Design review of the part built by this model. Coordinates are the model's own, in mm. Face numbers are marked on the shaded views. A direction names the side the tool comes from. Round coordinates to 2 decimals unless told otherwise and drop trailing zeros. Order: outer loops, then holes, each group sorted by start corner. A loop starts at its lowest first (then second) coordinate and runs counter-clockwise, first axis right, second up. Notation, with made-up numbers: (55, 56.5) - (66, 56.5) arc R23 ccw to (66, 91.5) - close; hole circle Ø3 at (42.5, 83.5). An arc over 180 degrees is marked (long way). Use CSV: the item, a comma, the result in double quotes.
from build123d import *

# Parameters (mm, degrees)
SKETCH1_W           = 105
SKETCH1_H           = 70
BOSS_EXTRUDE1_DEPTH = 10
SKETCH2_W           = 20
SKETCH2_H           = 70
BOSS_EXTRUDE2_DEPTH = 70
CUT_EXTRUDE1_DEPTH  = 20
SKETCH4_R           = 25.5
CUT_EXTRUDE2_DEPTH  = 10
SKETCH5_R           = 15.5
CUT_EXTRUDE3_DEPTH  = 4
SKETCH7_R           = 2.5
CUT_EXTRUDE5_DEPTH  = 10
SKETCH9_W           = 10
SKETCH9_H           = 70
BOSS_EXTRUDE4_DEPTH = 35
SKETCH10_R          = 19
CUT_EXTRUDE7_DEPTH  = 10
SKETCH11_R          = 2.5
CUT_EXTRUDE9_DEPTH  = 10
SKETCH6_R           = 12.5
CUT_EXTRUDE10_DEPTH = 10
SKETCH13_W          = 35
SKETCH13_H          = 35
CUT_EXTRUDE11_DEPTH = 10


with BuildPart() as part:
    # Sketch1 → Boss-Extrude1 (new body)
    with BuildSketch(Plane(origin=(0, 0, 0), x_dir=(1, 0, 0), z_dir=(0, 1, 0))):
        Rectangle(SKETCH1_W, SKETCH1_H)
    extrude(amount=BOSS_EXTRUDE1_DEPTH)

    # Sketch2 → Boss-Extrude2 (add)
    with BuildSketch(Plane(origin=(0, 10, 0), x_dir=(1, 0, 0), z_dir=(0, 1, 0))):
        with Locations((42.5, 0)):
            Rectangle(SKETCH2_W, SKETCH2_H)
    extrude(amount=BOSS_EXTRUDE2_DEPTH)

    # Sketch3 → Cut-Extrude1 (cut)
    with BuildSketch(Plane.ZY.offset(-32.5)):
        with BuildLine():
            Line((3e-08, 80), (-35, 80))
            Line((-35, 80), (-35, 45))
            ThreePointArc((-35, 45), (-24.748737331, 69.748737352), (3e-08, 80))
        make_face()
        with BuildLine():
            Line((35, 80), (3e-08, 80))
            ThreePointArc((3e-08, 80), (24.748737352, 69.748737331), (35, 45))
            Line((35, 45), (35, 80))
        make_face()
    extrude(amount=-CUT_EXTRUDE1_DEPTH, mode=Mode.SUBTRACT)

    # Sketch4 → Cut-Extrude2 (cut)
    with BuildSketch(Plane.ZY.offset(-32.5)):
        with Locations((0, 45)):
            Circle(SKETCH4_R)
    extrude(amount=-CUT_EXTRUDE2_DEPTH, mode=Mode.SUBTRACT)

    # Sketch5 → Cut-Extrude3 (cut)
    with BuildSketch(Plane.ZY.offset(-42.5)):
        with Locations((0, 45)):
            Circle(SKETCH5_R)
    extrude(amount=-CUT_EXTRUDE3_DEPTH, mode=Mode.SUBTRACT)

    # Sketch7 → Cut-Extrude5 (cut)
    with BuildSketch(Plane.ZY.offset(-42.5)):
        with Locations((14.142135624, 59.142135624)):
            Circle(SKETCH7_R)
        with Locations((14.142135624, 30.857864376)):
            Circle(SKETCH7_R)
        with Locations((-14.142135624, 30.857864376)):
            Circle(SKETCH7_R)
        with Locations((-14.142135624, 59.142135624)):
            Circle(SKETCH7_R)
    extrude(amount=-CUT_EXTRUDE5_DEPTH, mode=Mode.SUBTRACT)

    # Sketch9 → Boss-Extrude4 (add)
    with BuildSketch(Plane(origin=(0, 10, 0), x_dir=(1, 0, 0), z_dir=(0, 1, 0))):
        with Locations((-47.5, 0)):
            Rectangle(SKETCH9_W, SKETCH9_H)
    extrude(amount=BOSS_EXTRUDE4_DEPTH)

    # Sketch10 → Cut-Extrude7 (cut)
    with BuildSketch(Plane.ZY.offset(52.5)):
        with Locations((0, 45)):
            Circle(SKETCH10_R)
    extrude(amount=-CUT_EXTRUDE7_DEPTH, mode=Mode.SUBTRACT)

    # Sketch11 → Cut-Extrude9 (cut)
    with BuildSketch(Plane(origin=(0, 10, 0), x_dir=(1, 0, 0), z_dir=(0, 1, 0))):
        with Locations((-32.5, 25)):
            Circle(SKETCH11_R)
        with Locations((22.5, 25)):
            Circle(SKETCH11_R)
        with Locations((22.5, -25)):
            Circle(SKETCH11_R)
        with Locations((-32.5, -25)):
            Circle(SKETCH11_R)
    extrude(amount=-CUT_EXTRUDE9_DEPTH, mode=Mode.SUBTRACT)

    # Sketch6 → Cut-Extrude10 (cut)
    with BuildSketch(Plane.ZY.offset(-46.5)):
        with Locations((0, 45)):
            Circle(SKETCH6_R)
    extrude(amount=-CUT_EXTRUDE10_DEPTH, mode=Mode.SUBTRACT)

    # Sketch13 → Cut-Extrude11 (cut)
    with BuildSketch(Plane(origin=(0, 10, 0), x_dir=(1, 0, 0), z_dir=(0, 1, 0))):
        with Locations((-5, 0)):
            Rectangle(SKETCH13_W, SKETCH13_H)
    extrude(amount=-CUT_EXTRUDE11_DEPTH, mode=Mode.SUBTRACT)


solid = part.part
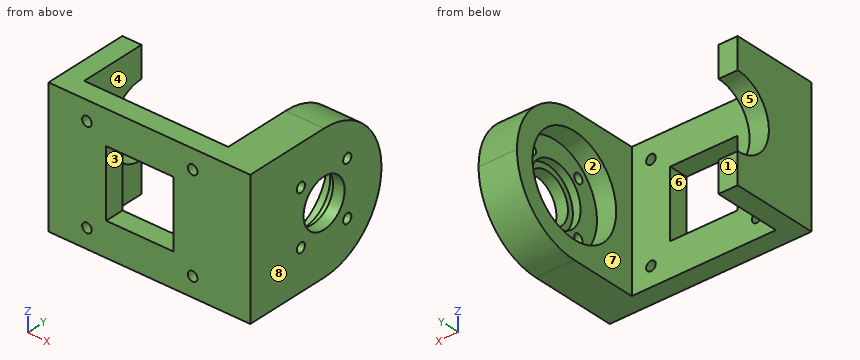
1) We need section B-B (x = -32.5). Give the boundary of the cut face in (y, z), then the cut area to 3 significant figures.
Data:
outline,"(0, -35) - (10, -35) - (10, -27.5) - (0, -27.5) - close; (0, -22.5) - (10, -22.5) - (10, 22.5) - (0, 22.5) - close; (0, 27.5) - (10, 27.5) - (10, 35) - (0, 35) - close"
area,"600 mm2"
2) Insertion check: pin 1 Ø1 at (x, z) = (22.5, 13) entering from +Y; pin 2 Ø15.5 at (y, z) = (37.5, -2.5) entering from -X; pin 3 Ø8 at (x, z) = (-50, -30.5) entering from +Y. Each pin has a flat end and moves straight along its axis. Give the tip position at first contact, or say it passes through.
Data:
pin 1,"stops at y = 10"
pin 2,"stops at x = 42.5"
pin 3,"stops at y = 45"
3) For the marked faces 1, 2, 3 and 4, list the 3-axis set-ups (+Z, -Z, +X, -X, +Y, -Y) from which the entire face can be reached by the end or side of a thin tool; tool diameter is ignored.
Data:
face 1,"+Z, -Z, -X, +Y"
face 2,"none"
face 3,"+Y, -Y"
face 4,"+Z, -Z, +Y"
4) We need section A-A (x = -18). Give the boundary of the cut face in (y, z).
Data:
outline,"(0, -35) - (10, -35) - (10, -17.5) - (0, -17.5) - close; (0, 17.5) - (10, 17.5) - (10, 35) - (0, 35) - close"
5) To check wall thickness, follow L1, parallel to X at y = 7.25, z = -25; L2, parallel to X at y = 9, z = 8; L3, parallel to X at y = 36, z = -25. State the ranges of each line that lie inside material, in increasing order. Write a range as from..to.
Data:
L1,"x = -52.5..-35, -30..20, 25..52.5"
L2,"x = -52.5..-22.5, 12.5..52.5"
L3,"x = -52.5..-42.5, 32.5..52.5"
6) We need section D-D (y = 40.5). Give the boundary of the cut face in (x, z).
Data:
outline,"(-52.5, -35) - (-42.5, -35) - (-42.5, -18.46) - (-52.5, -18.46) - close; (-52.5, 18.46) - (-42.5, 18.46) - (-42.5, 35) - (-52.5, 35) - close; (32.5, -35) - (52.5, -35) - (52.5, -11.66) - (46.5, -11.66) - (46.5, -14.83) - (42.5, -14.83) - (42.5, -25.1) - (32.5, -25.1) - close; (32.5, 25.1) - (42.5, 25.1) - (42.5, 14.83) - (46.5, 14.83) - (46.5, 11.66) - (52.5, 11.66) - (52.5, 35) - (32.5, 35) - close"
7) The part is to be moulded in two halves that separate along X. For the marked faces 5, 6, 7 and 8, say which applies: +X half, -X half, draft (parallel to the pull), parting line (faces both ways), or undercut.
Data:
face 5,"draft"
face 6,"undercut"
face 7,"undercut"
face 8,"+X half"
8) We need section C-C (z = 1.5). Give the boundary of the cut face in (x, y), then the cut area to 3 significant figures.
Data:
outline,"(-52.5, 0) - (-22.5, 0) - (-22.5, 10) - (-42.5, 10) - (-42.5, 26.06) - (-52.5, 26.06) - close; (12.5, 0) - (52.5, 0) - (52.5, 32.59) - (46.5, 32.59) - (46.5, 29.57) - (42.5, 29.57) - (42.5, 19.54) - (32.5, 19.54) - (32.5, 10) - (12.5, 10) - close; (32.5, 70.46) - (42.5, 70.46) - (42.5, 60.43) - (46.5, 60.43) - (46.5, 57.41) - (52.5, 57.41) - (52.5, 79.97) - (32.5, 79.97) - close"
area,"1,480 mm2"
